Geometry: final body of the model. Coordinates: model frame, mm. Face numbers are marked on the shaded views. Coordinates: 2 decimals unless noted, no trailing zeros. Write each loop counter-clockwise with the first axis right and the second up, starting at its lowest first coordinate (ties: lowest second). Pieces come first, ordered by that corner, then holes. Notation, with made-up numbers: (76.5, 7) -> (135.5, 7) arc R18 cw to (135.5, 22) -> close; hole circle Ø4 at (14.25, -34.75). An arc over 180 degrees is marked (long way). One line per item, written item: value.
```python
from build123d import *

# Parameters (mm, degrees)
BOSS_EXTRUDE1_DEPTH = 5
SKETCH4_R           = 1.5
CUT_EXTRUDE1_DEPTH  = 6
FILLET1_R           = 1.5


with BuildPart() as part:
    # Sketch2 → Boss-Extrude1 (new body)
    with BuildSketch(Plane.XY):
        with BuildLine():
            Line((8, 20.584180911), (2, 20.584180911))
            ThreePointArc((2, 20.584180911), (0.585786438, 19.998394474), (0, 18.584180911))
            Line((0, 18.584180911), (0, -25.915819089))
            ThreePointArc((0, -25.915819089), (0.585786438, -27.330032651), (2, -27.915819089))
            Line((2, -27.915819089), (8, -27.915819089))
            ThreePointArc((8, -27.915819089), (9.414213562, -27.330032651), (10, -25.915819089))
            Line((10, -25.915819089), (10, 18.584180911))
            ThreePointArc((10, 18.584180911), (9.414213562, 19.998394474), (8, 20.584180911))
        make_face()
    extrude(amount=BOSS_EXTRUDE1_DEPTH)

    # Sketch4 → Cut-Extrude1 (cut, through all)
    with BuildSketch(Plane(origin=(0, 0, 0), x_dir=(-1, 0, 0), z_dir=(0, 0, -1))):
        with Locations((-5, -23.915819089)):
            Circle(SKETCH4_R)
        with Locations((-5, 16.584180911)):
            Circle(SKETCH4_R)
    extrude(amount=-CUT_EXTRUDE1_DEPTH, mode=Mode.SUBTRACT)

    # Fillet1
    fillet1_edges = [part.edges().sort_by_distance(p)[0] for p in [
        (0.585786438, 19.998394474, 5),
        (0, -3.665819089, 5),
        (0.585786438, -27.330032651, 5),
        (5, -27.915819089, 5),
        (9.414213562, -27.330032651, 5),
        (10, -3.665819089, 5),
        (9.414213562, 19.998394474, 5),
        (5, 20.584180911, 5),
    ]]
    fillet(fillet1_edges, radius=FILLET1_R)


solid = part.part
```
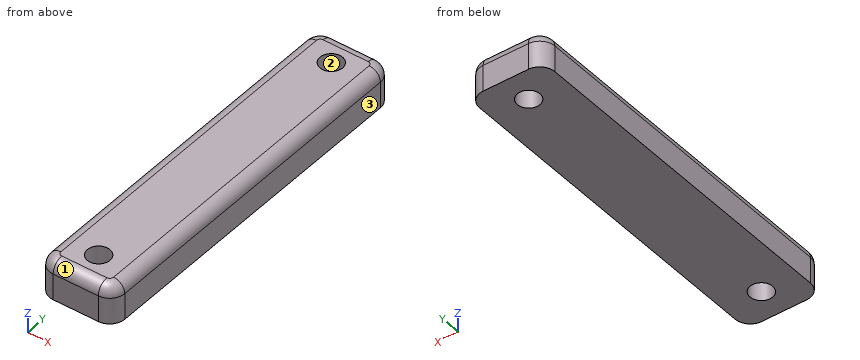
(1) Section C-C (y = -23.5). Return the cut outline in (x, z).
Responses:
outline: (0, 0) -> (3.56, 0) -> (3.56, 5) -> (1.5, 5) arc R1.5 ccw to (0, 3.5) -> close; (6.44, 0) -> (10, 0) -> (10, 3.5) arc R1.5 ccw to (8.5, 5) -> (6.44, 5) -> close
(2) Section D-D (y = 10.5). Return the cut outline in (x, z), then the cut area to 3 significant figures.
Responses:
outline: (0, 0) -> (10, 0) -> (10, 3.5) arc R1.5 ccw to (8.5, 5) -> (1.5, 5) arc R1.5 ccw to (0, 3.5) -> close
area: 49.0 mm2
(3) Section A-A (x = 5). Return the cut outline in (y, z).
Responses:
outline: (-27.92, 0) -> (-25.42, 0) -> (-25.42, 5) -> (-26.42, 5) arc R1.5 ccw to (-27.92, 3.5) -> close; (-22.42, 0) -> (15.08, 0) -> (15.08, 5) -> (-22.42, 5) -> close; (18.08, 0) -> (20.58, 0) -> (20.58, 3.5) arc R1.5 ccw to (19.08, 5) -> (18.08, 5) -> close
(4) Section B-B (z = 1.35). Return the cut outline in (x, y).
Responses:
outline: (0, -25.92) arc R2 ccw to (2, -27.92) -> (8, -27.92) arc R2 ccw to (10, -25.92) -> (10, 18.58) arc R2 ccw to (8, 20.58) -> (2, 20.58) arc R2 ccw to (0, 18.58) -> close; hole circle Ø3 at (5, -23.92); hole circle Ø3 at (5, 16.58)
(5) Pull-direction query (Y, two-part tool) for the marked faces 1, 2 and 3; classes: released by +Y, released by -Y, zero draft, split by the parting line, or undercut.
Responses:
face 1: released by -Y
face 2: undercut
face 3: zero draft
(6) Line query: line 1 (Y direction, x = 5, z = 3.2); line 2 (Y direction, x = 5.5, z = 2.2); line 3 (X direction, y = 6.5, z = 3.65). Output: solid intervals per line, ascending. Write a range as [from, to].
Responses:
line 1: y = [-27.92, -25.42], [-22.42, 15.08], [18.08, 20.58]
line 2: y = [-27.92, -25.33], [-22.5, 15.17], [18, 20.58]
line 3: x = [0.01, 9.99]
